Geometry check sheet. Reference: the model listing, model coordinates, mm. A direction names the side the tool comes from. Coordinates: 2 decimals unless noted, no trailing zeros. Loops run counter-clockwise (first coordinate to the right, second up) from the corner with the lowest first, then second, coordinate; pieces in that order, holes last. Notation, with made-up numbers: (69.5, -38.5) - (82.5, -38.5) arc R33 ccw to (82.5, -5.5) - close; hole circle Ø9 at (43, 21.25). An arc over 180 degrees is marked (long way). Write each question's results on one line, items separated by ' | '. Start each with the question number.
(1) Material ranges on probe 1 along Y at (x, z) = (0, -1.45); probe 2 along Y at (x, z) = (0, -0.7); probe 3 along X at (y, z) = (21, -0.2), recorded low to high.
(2) Sectioned sample at A-A (x = 0). Enter the section's corners in (y, z), plus the area to 3 significant figures.
(3) Sectioned sample at B-B (y = 0). Enter the section's corners in (x, z).
(4) Go/stop test with flat-tipped pins: pin 1 Ø2.5 at (x, y) = (1.5, 25) entering from +Z; pin 2 Ø1 at (y, z) = (8.5, -0.5) entering from +X. Record where each tip stops, or that it passes through.
(5) Access from +Z, -Z, +X, -X, +Y, -Y to the whole of each face (thin tool, end or side, straight path). Record for faces 5 (the face through (0, -6, -3)), 6 (the face through (0, -24, -2.8)).
(6) Mould release check, pull along Y, two halves, no side actions. Record for faces 1 (the face through (-1.45, 0.06, -1.48)), 2 (the face through (-29.97, 1.32, -1.5)), 3 (the face through (0, 24, -2.8)), 4 (the face through (0, -6, 0)): pulls with the +Y half, pulls with the -Y half, needs draft (parallel to the pull), parting line crosses it, or undercut.
Autodesk Fusion 360 part; units mm, degrees
sketch "Sketch1" plane through (0, 0, 0) normal (0, 0, 1) x (1, 0, 0)
  circle A0 centre (0, 0) radius 30
  circle A1 centre (0, 23.95) radius 4.05
  line L0 (-30, 0) -> (30, 0)
  circle A2 centre (0, -23.95) radius 4.05
  circle A3 centre (0, 0) radius 1.45
  dimension "d1" = 60
  dimension "d2" = 8.1
  dimension "d3" = 2
  dimension "d4" = 2.9
extrude "Extrude1" add sketch "Sketch1" against normal blind 3 contours A0 L0 A3 | A0 L0 A3 | A1 | A2
extrude "Extrude2" cut sketch "Sketch1" against normal blind 2.8 contours A1 | A2
chamfer "Chamfer1" distance 1.2 angle 45 2 edges at (-27.9698, -10.8485, 0) (-27.9698, 10.8485, -3)
chamfer "Chamfer2" distance 0.4 angle 45 2 edges at (-3.7759, -22.4855, 0) (-3.7759, 25.4145, 0)
Outcome:
1) probe 1: y = -30 to -28, -19.9 to -1.45, 1.45 to 19.9, 28 to 30 | probe 2: y = -29.5 to -28, -19.9 to -1.45, 1.45 to 19.9, 28 to 29.5 | probe 3: x = -20 to -3.06, 3.06 to 20
2) outline: (-30, -1.8) - (-28.8, -3) - (-1.45, -3) - (-1.45, 0) - (-19.5, 0) - (-19.9, -0.4) - (-19.9, -2.8) - (-28, -2.8) - (-28, -0.4) - (-28.4, 0) - (-28.8, 0) - (-30, -1.2) - close; (1.45, -3) - (28.8, -3) - (30, -1.8) - (30, -1.2) - (28.8, 0) - (28.4, 0) - (28, -0.4) - (28, -2.8) - (19.9, -2.8) - (19.9, -0.4) - (19.5, 0) - (1.45, 0) - close | area: 123 mm2
3) outline: (-30, -1.8) - (-28.8, -3) - (-1.45, -3) - (-1.45, 0) - (-28.8, 0) - (-30, -1.2) - close; (1.45, -3) - (28.8, -3) - (30, -1.8) - (30, -1.2) - (28.8, 0) - (1.45, 0) - close
4) pin 1: stops at z = -2.8 | pin 2: stops at x = 28.58
5) face 5: -Z, +X, -X, +Y, -Y | face 6: +Z
6) face 1: undercut | face 2: parting line crosses it | face 3: undercut | face 4: needs draft
